Check sheet for the modelled part. Datum: model origin and axes. Units: mm. Face numbers are marked on the shaded views. A direction names the side the tool comes from. Round coordinates to 2 decimals unless told otherwise and drop trailing zeros. Write each loop counter-clockwise with the first axis right and the second up, starting at its lowest first coordinate (ties: lowest second). Pieces come first, ordered by that corner, then holes. Notation, with made-up numbers: M -32.5,-19 L -3.5,-19 A35 ccw -3.5,18 Z; hole C 38.25,-0.75 d6. An arc over 180 degrees is marked long. One line per item, written item: value.
from build123d import *

# Parameters (mm, degrees)
EXTRUDE_THIN1_DEPTH                            = 37.5
SKETCH4_R                                      = 5.5
CUT_EXTRUDE1_DEPTH                             = 72.4375
CUT_EXTRUDE1_DEPTH_BACK                        = 5.7625
M5_CLEARANCE_HOLE1_D                           = 5.5
M6_CLEARANCE_HOLE2_D                           = 6.6
CSK_FOR_M3_FLAT_HEAD_MACHINE_SCREW1_AT_2_COUNT = 2
CSK_FOR_M3_FLAT_HEAD_MACHINE_SCREW1_AT_2_PITCH = 11.5
CSK_FOR_M3_FLAT_HEAD_MACHINE_SCREW1_AT_3_COUNT = 2
CSK_FOR_M3_FLAT_HEAD_MACHINE_SCREW1_AT_3_PITCH = 16.263455967
CSK_FOR_M3_FLAT_HEAD_MACHINE_SCREW1_AT_4_COUNT = 2
CSK_FOR_M3_FLAT_HEAD_MACHINE_SCREW1_AT_4_PITCH = 11.5
CSK_FOR_M3_SFHCS2_D                            = 3.4
CSK_FOR_M3_SFHCS2_DEPTH                        = 10
CSK_FOR_M3_SFHCS2_CSINK_D                      = 6.72
CSK_FOR_M3_SFHCS2_CSINK_ANGLE                  = 90
CSK_FOR_M3_SFHCS2_TIP                          = 1.021463052
M3_CLEARANCE_HOLE1_D                           = 3.4
M3X0_5_TAPPED_HOLE2_AT_2_COUNT                 = 2
M3X0_5_TAPPED_HOLE2_AT_2_PITCH                 = 65
M3X0_5_TAPPED_HOLE2_AT_3_COUNT                 = 2
M3X0_5_TAPPED_HOLE2_AT_3_PITCH                 = 76.321687612
M3X0_5_TAPPED_HOLE2_AT_4_COUNT                 = 2
M3X0_5_TAPPED_HOLE2_AT_4_PITCH                 = 40
M5_CLEARANCE_HOLE2_D                           = 5.5


with BuildPart() as part:
    # Sketch3 → Extrude-Thin1 (new body, symmetric)
    with BuildSketch(Plane(origin=(0, 0, 0), x_dir=(0, 0, -1), z_dir=(1, 0, 0))):
        Polygon((53, 0), (0, 0), (0, 76.2), (53, 76.2), (53, 71.4375), (4.7625, 71.4375), (4.7625, 4.7625), (53, 4.7625), align=None)
    extrude(amount=EXTRUDE_THIN1_DEPTH, both=True)

    # Sketch4 → Cut-Extrude1 (cut, two sides)
    with BuildSketch(Plane(origin=(0, 4.7625, 0), x_dir=(1, 0, 0), z_dir=(0, 1, 0))) as cut_extrude1_sk:
        with Locations((0, 31.7625)):
            Circle(SKETCH4_R)
    extrude(amount=CUT_EXTRUDE1_DEPTH, mode=Mode.SUBTRACT)
    extrude(cut_extrude1_sk.sketch, amount=-CUT_EXTRUDE1_DEPTH_BACK, mode=Mode.SUBTRACT)

    # M5 Clearance Hole1 (through all)
    with Locations(Plane.XY):
        with Locations((-26.5, 58.1005), (26.5, 58.1005), (26.5, 18.1005), (-26.5, 18.1005)):
            Hole(M5_CLEARANCE_HOLE1_D / 2)

    # M6 Clearance Hole2 (through all)
    with Locations(Plane(origin=(0, 0, 0), x_dir=(-1, 0, 0), z_dir=(0, -1, 0))):
        with Locations((30, 28), (-30, 28)):
            Hole(M6_CLEARANCE_HOLE2_D / 2)

    # Sketch11 → CSK for M3 Flat Head Machine Screw1 (revolve, cut)
    with BuildSketch(Plane(origin=(-5.75, 0, -26.0125), x_dir=(0, 0, -1), z_dir=(1, 0, 0))):
        Polygon((0, 0), (0, 11.021463052), (1.7, 10), (1.7, 1.45), (3.15, 0), align=None)
    csk_for_m3_flat_head_machine_screw1 = revolve(axis=Axis((-5.75, -6.35, -26.0125), (0, 1, 0)), mode=Mode.SUBTRACT)

    # CSK for M3 Flat Head Machine Screw1 at 2: CSK for M3 Flat Head Machine Screw1 ×2
    with Locations(*[(i * CSK_FOR_M3_FLAT_HEAD_MACHINE_SCREW1_AT_2_PITCH, 0, 0) for i in range(1, CSK_FOR_M3_FLAT_HEAD_MACHINE_SCREW1_AT_2_COUNT)]):
        add(csk_for_m3_flat_head_machine_screw1, mode=Mode.SUBTRACT)

    # CSK for M3 Flat Head Machine Screw1 at 3: CSK for M3 Flat Head Machine Screw1 ×2
    with Locations(*[Vector(0.707106781, 0, -0.707106781) * (i * CSK_FOR_M3_FLAT_HEAD_MACHINE_SCREW1_AT_3_PITCH) for i in range(1, CSK_FOR_M3_FLAT_HEAD_MACHINE_SCREW1_AT_3_COUNT)]):
        add(csk_for_m3_flat_head_machine_screw1, mode=Mode.SUBTRACT)

    # CSK for M3 Flat Head Machine Screw1 at 4: CSK for M3 Flat Head Machine Screw1 ×2
    with Locations(*[(0, 0, -i * CSK_FOR_M3_FLAT_HEAD_MACHINE_SCREW1_AT_4_PITCH) for i in range(1, CSK_FOR_M3_FLAT_HEAD_MACHINE_SCREW1_AT_4_COUNT)]):
        add(csk_for_m3_flat_head_machine_screw1, mode=Mode.SUBTRACT)

    # Mirror1: CSK for M3 Flat Head Machine Screw1 across plane
    add(csk_for_m3_flat_head_machine_screw1.mirror(Plane(origin=(0, 38.1, 0), x_dir=(0, 0, 1), z_dir=(0, -1, 0))), mode=Mode.SUBTRACT)

    # Mirror1 copy 1 sketch → Mirror1 copy 1 (revolve, cut)
    with BuildSketch(Plane(origin=(5.75, 76.2, -26.0125), x_dir=(0, 0, -1), z_dir=(1, 0, 0))):
        Polygon((0, 0), (0, -11.021463052), (1.7, -10), (1.7, -1.45), (3.15, 0), align=None)
    revolve(axis=Axis((5.75, 82.55, -26.0125), (0, 1, 0)), mode=Mode.SUBTRACT)

    # Mirror1 copy 2 sketch → Mirror1 copy 2 (revolve, cut)
    with BuildSketch(Plane(origin=(5.75, 76.2, -37.5125), x_dir=(0, 0, -1), z_dir=(1, 0, 0))):
        Polygon((0, 0), (0, -11.021463052), (1.7, -10), (1.7, -1.45), (3.15, 0), align=None)
    revolve(axis=Axis((5.75, 82.55, -37.5125), (0, 1, 0)), mode=Mode.SUBTRACT)

    # Mirror1 copy 3 sketch → Mirror1 copy 3 (revolve, cut)
    with BuildSketch(Plane(origin=(-5.75, 76.2, -37.5125), x_dir=(0, 0, -1), z_dir=(1, 0, 0))):
        Polygon((0, 0), (0, -11.021463052), (1.7, -10), (1.7, -1.45), (3.15, 0), align=None)
    revolve(axis=Axis((-5.75, 82.55, -37.5125), (0, 1, 0)), mode=Mode.SUBTRACT)

    # CSK for M3 SFHCS2
    with Locations(Plane(origin=(0, 71.4375, 0), x_dir=(-1, 0, 0), z_dir=(0, -1, 0))):
        with Locations((15.5, 47.2625), (15.5, 16.2625), (-15.5, 16.2625), (-15.5, 47.2625)):
            CounterSinkHole(CSK_FOR_M3_SFHCS2_D / 2, CSK_FOR_M3_SFHCS2_CSINK_D / 2, depth=CSK_FOR_M3_SFHCS2_DEPTH, counter_sink_angle=CSK_FOR_M3_SFHCS2_CSINK_ANGLE)
            with Locations((0, 0, -(CSK_FOR_M3_SFHCS2_DEPTH + CSK_FOR_M3_SFHCS2_TIP / 2))):  # 118° drill point
                Cone(0, CSK_FOR_M3_SFHCS2_D / 2, CSK_FOR_M3_SFHCS2_TIP, mode=Mode.SUBTRACT)

    # M3 Clearance Hole1 (through all)
    with Locations(Plane(origin=(0, 76.2, 0), x_dir=(1, 0, 0), z_dir=(0, 1, 0))):
        with Locations((-15.5, 47.2625), (15.5, 47.2625), (15.5, 16.2625), (-15.5, 16.2625)):
            Hole(M3_CLEARANCE_HOLE1_D / 2)

    # Sketch19 → M3x0.5 Tapped Hole2 (revolve, cut)
    with BuildSketch(Plane(origin=(-32.5, 76.2, -48), x_dir=(0, 0, 1), z_dir=(1, 0, 0))):
        Polygon((0, 0), (0, 8.251075774), (1.25, 7.5), (1.25, 0), align=None)
    m3x0_5_tapped_hole2 = revolve(axis=Axis((-32.5, 82.55, -48), (0, -1, 0)), mode=Mode.SUBTRACT)

    # M3x0.5 Tapped Hole2 at 2: M3x0.5 Tapped Hole2 ×2
    with Locations(*[(i * M3X0_5_TAPPED_HOLE2_AT_2_PITCH, 0, 0) for i in range(1, M3X0_5_TAPPED_HOLE2_AT_2_COUNT)]):
        add(m3x0_5_tapped_hole2, mode=Mode.SUBTRACT)

    # M3x0.5 Tapped Hole2 at 3: M3x0.5 Tapped Hole2 ×2
    with Locations(*[Vector(0.851658317, 0, 0.524097426) * (i * M3X0_5_TAPPED_HOLE2_AT_3_PITCH) for i in range(1, M3X0_5_TAPPED_HOLE2_AT_3_COUNT)]):
        add(m3x0_5_tapped_hole2, mode=Mode.SUBTRACT)

    # M3x0.5 Tapped Hole2 at 4: M3x0.5 Tapped Hole2 ×2
    with Locations(*[(0, 0, i * M3X0_5_TAPPED_HOLE2_AT_4_PITCH) for i in range(1, M3X0_5_TAPPED_HOLE2_AT_4_COUNT)]):
        add(m3x0_5_tapped_hole2, mode=Mode.SUBTRACT)

    # Mirror2: M3x0.5 Tapped Hole2 across plane
    add(m3x0_5_tapped_hole2.mirror(Plane(origin=(0, 38.1, 0), x_dir=(0, 0, 1), z_dir=(0, -1, 0))), mode=Mode.SUBTRACT)

    # Mirror2 copy 1 sketch → Mirror2 copy 1 (revolve, cut)
    with BuildSketch(Plane(origin=(32.5, 0, -48), x_dir=(0, 0, 1), z_dir=(1, 0, 0))):
        Polygon((0, 0), (0, -8.251075774), (1.25, -7.5), (1.25, 0), align=None)
    revolve(axis=Axis((32.5, -6.35, -48), (0, -1, 0)), mode=Mode.SUBTRACT)

    # Mirror2 copy 2 sketch → Mirror2 copy 2 (revolve, cut)
    with BuildSketch(Plane(origin=(32.5, 0, -8), x_dir=(0, 0, 1), z_dir=(1, 0, 0))):
        Polygon((0, 0), (0, -8.251075774), (1.25, -7.5), (1.25, 0), align=None)
    revolve(axis=Axis((32.5, -6.35, -8), (0, -1, 0)), mode=Mode.SUBTRACT)

    # Mirror2 copy 3 sketch → Mirror2 copy 3 (revolve, cut)
    with BuildSketch(Plane(origin=(-32.5, 0, -8), x_dir=(0, 0, 1), z_dir=(1, 0, 0))):
        Polygon((0, 0), (0, -8.251075774), (1.25, -7.5), (1.25, 0), align=None)
    revolve(axis=Axis((-32.5, -6.35, -8), (0, -1, 0)), mode=Mode.SUBTRACT)

    # M5 Clearance Hole2 (through all)
    with Locations(Plane.XY):
        with Locations((-9.175, 18.1), (-9.175, 58.1), (9.175, 58.1), (9.175, 18.1)):
            Hole(M5_CLEARANCE_HOLE2_D / 2)


solid = part.part
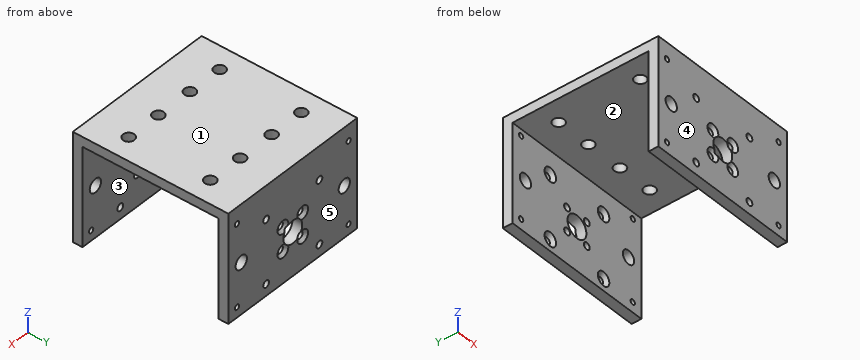
Q1. Draft check along Y on the marked faces 3, 4 and 5. Enter one of: pulls with the +Y half, pulls with the -Y half, needs draft (parallel to the pull), parting line crosses it, or undercut.
Completed:
face 3: undercut
face 4: pulls with the -Y half
face 5: pulls with the +Y half
Q2. Scan lines: line 1 (Z direction, x = 5.75, y = 72.7); line 2 (X direction, y = 58, z = -2); line 3 (Y direction, x = 6, z = -14). Record each from-to range of solid material in increasing order. Write a range as [from, to].
Completed:
line 1: [-53, -39.21], [-35.81, -27.71], [-24.31, 0]
line 2: [-37.5, -29.25], [-23.75, -11.92], [-6.43, 6.43], [11.92, 23.75], [29.25, 37.5]
line 3: [0, 4.76], [71.44, 76.2]
Q3. Sectioned sample at A-A on z = -8. Enter the section's corners in (x, y).
Completed:
outline: M -37.5,0 L -33.75,0 L -33.75,4.76 L -37.5,4.76 Z; M -37.5,71.44 L -33.75,71.44 L -33.75,76.2 L -37.5,76.2 Z; M -31.25,0 L 31.25,0 L 31.25,4.76 L -31.25,4.76 Z; M -31.25,71.44 L 31.25,71.44 L 31.25,76.2 L -31.25,76.2 Z; M 33.75,0 L 37.5,0 L 37.5,4.76 L 33.75,4.76 Z; M 33.75,71.44 L 37.5,71.44 L 37.5,76.2 L 33.75,76.2 Z
Q4. Sectioned sample at B-B on x = -15.5. Enter the section's corners in (y, z).
Completed:
outline: M 0,-53 L 4.76,-53 L 4.76,-48.96 L 0,-48.96 Z; M 0,-45.56 L 4.76,-45.56 L 4.76,-17.96 L 0,-17.96 Z; M 0,-14.56 L 4.76,-14.56 L 4.76,-4.76 L 71.44,-4.76 L 71.44,-12.9 L 73.1,-14.56 L 76.2,-14.56 L 76.2,0 L 0,0 Z; M 71.44,-53 L 76.2,-53 L 76.2,-48.96 L 73.1,-48.96 L 71.44,-50.62 Z; M 71.44,-43.9 L 73.1,-45.56 L 76.2,-45.56 L 76.2,-17.96 L 73.1,-17.96 L 71.44,-19.62 Z
Q5. Sectioned sample at C-C on z = -21.5. Enter the section's corners in (x, y), and give its area (3 significant figures).
Completed:
outline: M -37.5,0 L 37.5,0 L 37.5,4.76 L -37.5,4.76 Z; M -37.5,71.44 L 37.5,71.44 L 37.5,76.2 L -37.5,76.2 Z
area: 714 mm^2
Q6. Sectioned sample at D-D on y = 39. Enter the section's corners in (x, z).
Completed:
outline: M -37.5,-4.76 L 37.5,-4.76 L 37.5,0 L -37.5,0 Z
Q7. Access from +Z, -Z, +X, -X, +Y, -Y to the whole of each face (thin tool, end or side, straight path). Record for the marked faces 1 and 2.
Completed:
face 1: +Z, +X, -X, +Y, -Y
face 2: -Z, +X, -X
Q8. Depth check by flat-ended pin: P1, Ø4.5, axis at x = 5.75, z = -37.51, coming from the -Y side; P2, Ø7, axis at x = 26.5, y = 18.1, coming from the -Z side; P3, Ø5.5, axis at x = -5.75, z = -37.51, coming from the -Y side. Enter the tip coordinate at first touch or a pass-through.
Completed:
P1: y = 0.9
P2: z = -4.76
P3: y = 0.4
